from build123d import *

# Parameters (mm, degrees)
F0_W     = 127
F0_H     = 127
F0_W_2   = 113.03
F0_H_2   = 113.03
F1_DEPTH = 38.1
F2_W     = 113.03
F2_H     = 113.03
F3_DEPTH = 12.7
F4_R     = 5.08
F5_W     = 116.84
F5_H     = 116.84
F5_W_2   = 113.03
F5_H_2   = 113.03
F6_DEPTH = 12.7
F7_R     = 5.08


with BuildPart() as f1:
    # F0 (on Top) → F1 (new body)
    with BuildSketch(Plane.XY):
        Rectangle(F0_W, F0_H)
        Rectangle(F0_W_2, F0_H_2, mode=Mode.SUBTRACT)
    extrude(amount=F1_DEPTH)

    # F2 (on Top) → F3 (join)
    with BuildSketch(Plane.XY):
        Rectangle(F2_W, F2_H)
    extrude(amount=F3_DEPTH)

    # F4
    f4_edges = [f1.edges().sort_by_distance(p)[0] for p in [
        (-63.5, -63.5, 19.05),
        (-63.5, 63.5, 19.05),
        (63.5, 63.5, 19.05),
        (63.5, -63.5, 19.05),
    ]]
    fillet(f4_edges, radius=F4_R)

    # F5 (on face) → F6 (join)
    with BuildSketch(Plane.XY.offset(38.1)):
        Rectangle(F5_W, F5_H)
        Rectangle(F5_W_2, F5_H_2, mode=Mode.SUBTRACT)
    extrude(amount=F6_DEPTH)

    # F7
    f7_edges = [f1.edges().sort_by_distance(p)[0] for p in [
        (-58.42, -58.42, 44.45),
        (58.42, -58.42, 44.45),
        (58.42, 58.42, 44.45),
        (-58.42, 58.42, 44.45),
    ]]
    fillet(f7_edges, radius=F7_R)


solid = f1.part
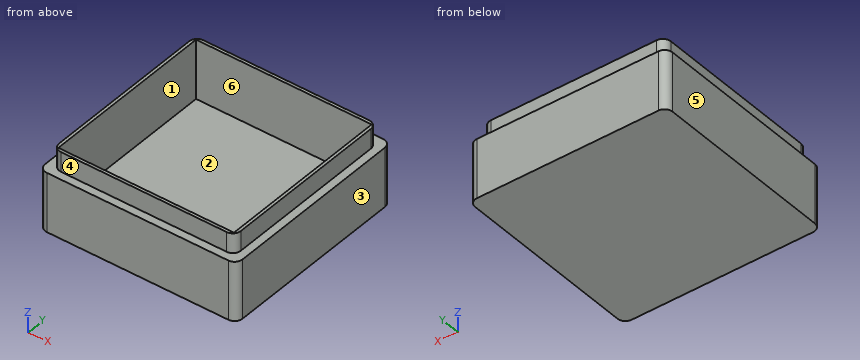
Could you check a few things on this model? Use its own coordinates, in mm. Face numbers are marked on the shaded views. A direction names the side the tool comes from. Give positions to 0.01 mm unless a question says otherwise; leave off trailing zeros. Order: outer loops, then holes, each group sorted by start corner. A loop starts at its lowest first (then second) coordinate and runs counter-clockwise, first axis right, second up. Notation, with made-up numbers: (-17.5, 5.25) -> (2.5, 5.25) arc R24 cw to (2.5, 19.25) -> close; hole circle Ø1 at (-3, -5). An arc over 180 degrees is marked (long way). Return JSON: item names as keys, results as strings.
1. Thinking about a two-plate mould opening in Y: for the marked faces 1, 2, 3 and 4, which applies, pulls with the +Y half, pulls with the -Y half, needs draft (parallel to the pull), parting line crosses it, or undercut?
Answer list:
{"face 1": "undercut", "face 2": "undercut", "face 3": "needs draft", "face 4": "pulls with the -Y half"}
2. For pin 1 Ø4 at (y, z) = (-15.5, 42.5) entering from +X; pin 2 Ø4 at (y, z) = (20, 46.5) entering from -X; pin 3 Ø6.5 at (x, z) = (-18.5, 47) entering from -Y, each with a flat end and sliding along its axis, tell me the tip position at first contact or that it passes through.
Answer list:
{"pin 1": "stops at x = 58.42", "pin 2": "stops at x = -58.42", "pin 3": "stops at y = -58.42"}
3. Imagine slicing it at D-D on z = 17. List the corners of the cut face in (x, y) for me (3 decimals), then the cut area to 3 significant figures.
Answer list:
{"outline": "(-63.5, -58.42) arc R5.08 ccw to (-58.42, -63.5) -> (58.42, -63.5) arc R5.08 ccw to (63.5, -58.42) -> (63.5, 58.42) arc R5.08 ccw to (58.42, 63.5) -> (-58.42, 63.5) arc R5.08 ccw to (-63.5, 58.42) -> close; hole (-56.515, -56.515) -> (56.515, -56.515) -> (56.515, 56.515) -> (-56.515, 56.515) -> close", "area": "3,330 mm2"}
4. Imagine slicing it at A-A on y = 29.5. List the corners of the cut face in (x, z) for me (3 decimals), then the cut area to 3 significant figures.
Answer list:
{"outline": "(-63.5, 0) -> (63.5, 0) -> (63.5, 38.1) -> (58.42, 38.1) -> (58.42, 50.8) -> (56.515, 50.8) -> (56.515, 12.7) -> (-56.515, 12.7) -> (-56.515, 50.8) -> (-58.42, 50.8) -> (-58.42, 38.1) -> (-63.5, 38.1) -> close", "area": "2,020 mm2"}
5. Imagine slicing it at B-B on z = 40. List the corners of the cut face in (x, y) for me (3 decimals), then the cut area to 3 significant figures.
Answer list:
{"outline": "(-58.42, -53.34) arc R5.08 ccw to (-53.34, -58.42) -> (53.34, -58.42) arc R5.08 ccw to (58.42, -53.34) -> (58.42, 53.34) arc R5.08 ccw to (53.34, 58.42) -> (-53.34, 58.42) arc R5.08 ccw to (-58.42, 53.34) -> close; hole (-56.515, -56.515) -> (56.515, -56.515) -> (56.515, 56.515) -> (-56.515, 56.515) -> close", "area": "854 mm2"}
6. On a 3-axis mill with a long thin cutter (end or side, diameter ignored), from which of +Z, -Z, +X, -X, +Y, -Y can I reach the whole of each face in a straight line? I mean the marked faces 5 and 6. Say none if no direction works.
Answer list:
{"face 5": "+Z, -Z, -X, +Y, -Y", "face 6": "+Z"}
7. I need wall thicknesses on line 1 (X direction, y = 40, z = 37) (3 decimals); line 2 (Y direction, x = 43.5, z = 49) (3 decimals). Which ranges of each line are inside material? Lowest first, please. Write a range as from..to.
Answer list:
{"line 1": "x = -63.5..-56.515, 56.515..63.5", "line 2": "y = -58.42..-56.515, 56.515..58.42"}
